from build123d import *

# Parameters (mm, degrees)
F0_W     = 1.266345
F0_H     = 6.32021
F0_W_2   = 2.438912
F0_H_2   = 7.262094
F0_W_3   = 3.07266
F0_H_3   = 10.11271
F1_DEPTH = 25.4


with BuildPart() as f1:
    # F0 (on Front) → F1 (new body)
    with BuildSketch(Plane.XZ):
        with BuildLine():
            ThreePointArc((79.519914, 39.215297), (91.139261, 27.59595), (79.519914, 15.976603))
            Line((79.519914, 15.976603), (55.234976, 15.976603))
            Line((55.234976, 15.976603), (47.973033, 15.976603))
            Line((47.973033, 15.976603), (47.973033, 9.44072))
            Line((47.973033, 9.44072), (55.234976, 9.44072))
            Line((55.234976, 9.44072), (79.519914, 9.44072))
            ThreePointArc((79.519914, 9.44072), (96.123763, 19.758998), (94.224531, 39.215297))
            ThreePointArc((94.224531, 39.215297), (87.719972, 44.562904), (79.519914, 46.477391))
            Line((79.519914, 46.477391), (63.599461, 46.477391))
            Line((63.599461, 46.477391), (62.705725, 46.477391))
            Line((62.705725, 46.477391), (55.234976, 46.477391))
            Line((55.234976, 46.477391), (47.973033, 46.477391))
            Line((47.973033, 46.477391), (47.973033, 39.215297))
            Line((47.973033, 39.215297), (55.234976, 39.215297))
            Line((55.234976, 39.215297), (79.519914, 39.215297))
        make_face()
        Polygon((47.973033, 9.44072), (47.973033, 15.976603), (47.973033, 39.215297), (47.973033, 46.477391), (44.974909, 46.477391), (43.708564, 46.477391), (40.711089, 46.477391), (40.711089, 3.812549), (47.973033, 3.812549), align=None)
        with Locations((44.341736, 49.637496)):
            Rectangle(F0_W, F0_H)
        Polygon((33.449145, 3.812549), (40.711089, 3.812549), (40.711089, 46.477391), (37.713614, 46.477391), (36.447269, 46.477391), (33.449145, 46.477391), align=None)
        with BuildLine():
            ThreePointArc((62.705725, 51.111013), (63.599461, 48.794202), (62.705725, 46.477391))
            Line((62.705725, 46.477391), (63.599461, 46.477391))
            ThreePointArc((63.599461, 46.477391), (64.326918, 49.020706), (62.705725, 51.111013))
        make_face()
        Polygon((43.708564, 52.797601), (44.974909, 52.797601), (46.24451, 52.797601), (46.24451, 54.079618), (44.974909, 54.079618), (43.708564, 54.079618), (42.431599, 54.079618), (42.431599, 52.797601), align=None)
        Polygon((26.187202, 3.812549), (33.449145, 3.812549), (33.449145, 46.477391), (30.451022, 46.477391), (29.818174, 46.477391), (29.184677, 46.477391), (26.187202, 46.477391), (26.187202, 39.215297), (26.187202, 15.976603), (26.187202, 9.44072), align=None)
        with BuildLine():
            ThreePointArc((79.519914, 46.477391), (87.719972, 44.562904), (94.224531, 39.215297))
            Line((94.224531, 39.215297), (115.830371, 39.215297))
            ThreePointArc((115.830371, 39.215297), (141.221769, 32.667561), (160.280371, 14.657407))
            Line((160.280371, 14.657407), (160.280371, 39.215297))
            Line((160.280371, 39.215297), (160.280371, 42.846344))
            Line((160.280371, 42.846344), (160.280371, 46.477391))
            Line((160.280371, 46.477391), (160.280371, 57.156805))
            Line((160.280371, 57.156805), (160.280371, 71.035281))
            ThreePointArc((160.280371, 71.035281), (141.221769, 53.025126), (115.830371, 46.477391))
            Line((115.830371, 46.477391), (79.519914, 46.477391))
        make_face()
        with Locations((37.080441, 49.637496)):
            Rectangle(F0_W, F0_H)
        Polygon((36.447269, 52.797601), (37.713614, 52.797601), (38.990579, 52.797601), (38.990579, 54.079618), (37.713614, 54.079618), (36.447269, 54.079618), (35.177668, 54.079618), (35.177668, 52.797601), align=None)
        Polygon((29.818174, 46.477391), (30.451022, 46.477391), (30.451022, 52.797601), (29.184677, 52.797601), (29.184677, 46.477391), align=None)
        with BuildLine():
            Line((0, 9.44072), (26.187202, 9.44072))
            Line((26.187202, 9.44072), (26.187202, 15.976603))
            Line((26.187202, 15.976603), (0, 15.976603))
            ThreePointArc((0, 15.976603), (-11.619347, 27.59595), (0, 39.215297))
            Line((0, 39.215297), (26.187202, 39.215297))
            Line((26.187202, 39.215297), (26.187202, 46.477391))
            Line((26.187202, 46.477391), (0, 46.477391))
            ThreePointArc((0, 46.477391), (-8.200058, 44.562904), (-14.704617, 39.215297))
            ThreePointArc((-14.704617, 39.215297), (-16.603849, 19.758998), (0, 9.44072))
        make_face()
        Polygon((29.184677, 52.797601), (30.451022, 52.797601), (31.720623, 52.797601), (31.720623, 54.079618), (30.451022, 54.079618), (29.184677, 54.079618), (27.907712, 54.079618), (27.907712, 52.797601), align=None)
        with BuildLine():
            Line((-37.184769, 39.215297), (-14.704617, 39.215297))
            ThreePointArc((-14.704617, 39.215297), (-8.200058, 44.562904), (0, 46.477391))
            Line((0, 46.477391), (-37.184769, 46.477391))
            Line((-37.184769, 46.477391), (-37.184769, 39.215297))
        make_face()
        with Locations((-38.404225, 42.846344)):
            Rectangle(F0_W_2, F0_H_2)
        Polygon((-42.769502, 37.789989), (-39.623681, 39.215297), (-39.623681, 46.477391), (-42.769502, 47.902699), align=None)
        with Locations((-44.305832, 42.846344)):
            Rectangle(F0_W_3, F0_H_3)
    extrude(amount=F1_DEPTH)


solid = f1.part
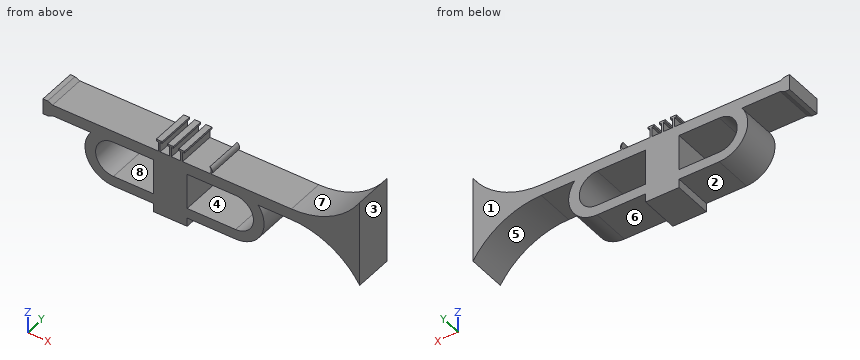
Could you check a few things on this model? Use its own coordinates, in mm. Face numbers are marked on the shaded views. A direction names the side the tool comes from. Give positions to 0.01 mm unless a question says otherwise; leave off trailing zeros. Write each loop counter-clockwise with the first axis right and the second up, starting at its lowest first coordinate (ties: lowest second). Pieces come first, ordered by that corner, then holes. Notation, with made-up numbers: (48.5, 1.5) -> (65.5, 1.5) arc R23 ccw to (65.5, 14.5) -> close; hole circle Ø8 at (80.5, 81). An arc over 180 degrees is marked (long way). Answer as CSV lines item,"result". Start each with the question number.
(1) If we section it at B-B, the plane z = 27: Write out the boundary of the cut face in (x, y).
(2) If we section it at D-D, the plane x = 135: Write out the boundary of the cut face in (y, z), and give its area (3 significant figures).
(3) Please list where these lines run through material, in increasing order: line 1 (Z direction, x = 24.5, y = -17); line 2 (X direction, y = -18, z = 22); line 3 (X direction, y = -15.75, z = 26).
(4) I'm going to push flat-ended pins straight in: pin 1 Ø1.5 at (x, y) = (-44.5, -14) entering from +Z; pin 2 Ø2 at (x, z) = (-15.5, 16) entering from -Y; pin 3 Ø6 at (x, y) = (40, -5.5) entering from +Z; pin 4 Ø1.4 at (y, z) = (-11.5, 53.5) entering from -X. Where does each tip first touch, or does it pass through?
(5) If we section it at C-C, the plane y = -4: Give the number of separate pieces and of enclosed holes in the cut face, and give its area (3 significant figures).
(6) If we section it at A-A, the plane x = 57: Write out the boundary of the cut face in (y, z), and give its area (3 significant figures).
(7) Which directions (+Z, -Z, +X, -X, +Y, -Y) give clear straight access to the entire face, cutting with the end or side of a thin tool? Please do the marked faces 1, 2, 3, 4 and 5.
(8) If we mould it in two halves opening along Z, with no side actions, what happens to the marked faces 6, 7 and 8? For each: +Z half, -Z half, draft (parallel to the pull), parting line (faces both ways), or undercut.
Answer list:
1,outline,"(-18.49, -25.4) -> (-11.6, -25.4) -> (-11.6, 0) -> (-18.49, 0) -> close; (26.19, -25.4) -> (47.97, -25.4) -> (47.97, 0) -> (26.19, 0) -> close; (91.12, -25.4) -> (98.01, -25.4) -> (98.01, 0) -> (91.12, 0) -> close; (149.5, -25.4) -> (160.28, -25.4) -> (160.28, 0) -> (149.5, 0) -> close"
2,outline,"(-25.4, 35.59) -> (0, 35.59) -> (0, 50.1) -> (-25.4, 50.1) -> close"
2,area,"369 mm^2"
3,line 1,"9.44 to 15.98, 39.22 to 46.48"
3,line 2,"-17.53 to -10.18, 26.19 to 47.97, 89.7 to 97.05, 154.71 to 160.28"
3,line 3,"-18.41 to -11.51, 26.19 to 47.97, 91.03 to 97.93, 150.66 to 160.28"
4,pin 1,"z = 47.9"
4,pin 2,"through"
4,pin 3,"z = 54.08"
4,pin 4,"x = 27.91"
5,separate pieces,"1"
5,enclosed holes,"2"
5,area,"3,850 mm^2"
6,outline,"(-25.4, 9.44) -> (0, 9.44) -> (0, 15.98) -> (-25.4, 15.98) -> close; (-25.4, 39.22) -> (0, 39.22) -> (0, 46.48) -> (-25.4, 46.48) -> close"
6,area,"350 mm^2"
7,face 1,"+Z, -Z, +X, -X, +Y"
7,face 2,"-Z, -X, +Y, -Y"
7,face 3,"+Z, -Z, +X, +Y, -Y"
7,face 4,"+Y, -Y"
7,face 5,"-Z, +Y, -Y"
8,face 6,"-Z half"
8,face 7,"+Z half"
8,face 8,"undercut"
